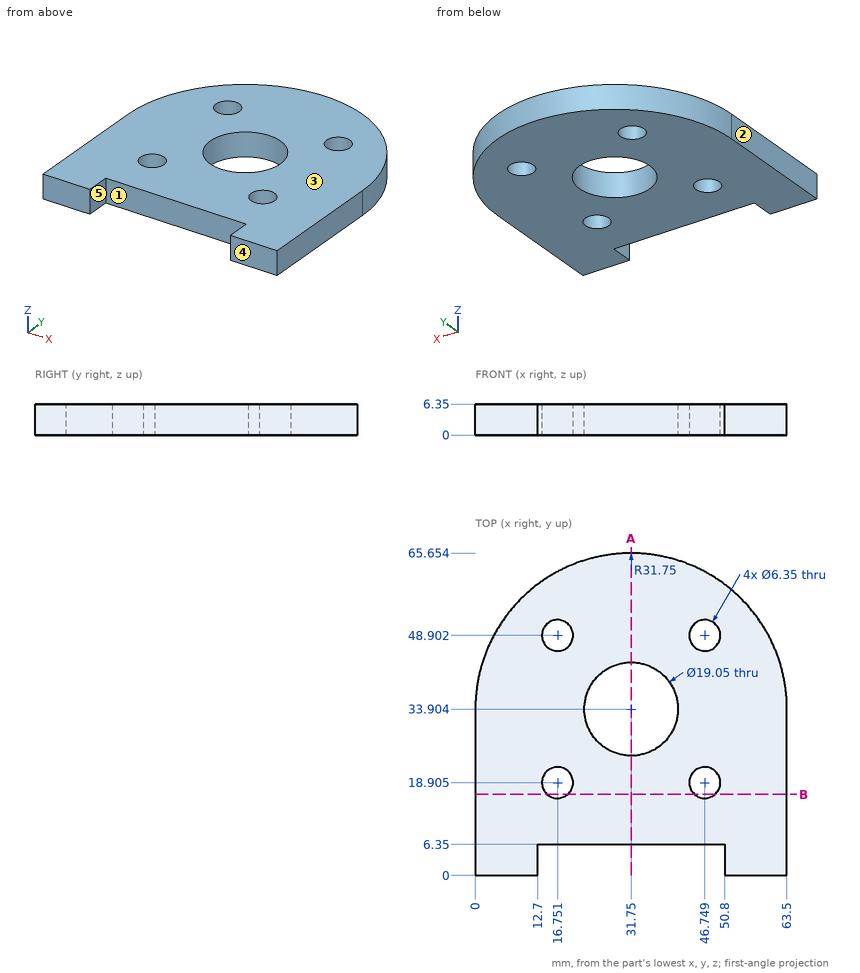
Answer from the drawing. Dimensions are ordinates in mm from the lowest x, y and z of the part. A direction names the side the tool comes from. Round coordinates to 2 decimals unless told otherwise and drop trailing zeros. Order: outer loops, then holes, each group sorted by start corner. A loop starts at its lowest first (then second) coordinate and runs counter-clockwise, first axis right, second up. Notation, with made-up numbers: (-3.5, 33) - (4.5, 33) arc R16 ccw to (4.5, 61) - close; hole circle Ø4 at (-7.75, -37.75). An arc over 180 degrees is marked (long way). Put each result on its own line as item: value. Start each with the question number.
(1) For the marked faces 4 and 5, determine the directions among +Z, -Z, +X, -X, +Y, -Y from which every point of the face is accessible in a straight line to the end or side of a thin tool.
(2) Determine the mould class of the marked faces 1, 2 and 3 for opening direction X: released by +X, released by -X, zero draft, split by the parting line, or undercut.
(3) Straight lines are drawn through the part: probe 1 along X at (y, z) = (3.5, 5.25); probe 2 along X at (y, z) = (29, 6) (1 decimal); probe 3 along Y at (x, z) = (55, 4) (1 decimal). For each, find the intervals that lie inside material, in ascending order. Write a range as from..to.
(4) Find section A-A (x = 31.75). Give the vertices of the cut face in (y, z), plus the area to 3 significant figures.
(5) Given P1, Ø17, axis at x = 31.75, y = 33.9, coming from the -Z side, flat-ended and moving along its own axis, determine where the tip first touches the part or whether it passes through.
(6) Find section B-B (y = 16.5). State how many separate pieces and enclosed holes the cut face has.
Reply:
1. face 4: +Z, -Z, +X, -X, -Y
1. face 5: +Z, -Z, -Y
2. face 1: undercut
2. face 2: released by -X
2. face 3: zero draft
3. probe 1: 0..12.7, 50.8..63.5
3. probe 2: 0..23.6, 39.9..63.5
3. probe 3: 0..55.5
4. outline: (6.35, 0) - (24.38, 0) - (24.38, 6.35) - (6.35, 6.35) - close; (43.43, 0) - (65.65, 0) - (65.65, 6.35) - (43.43, 6.35) - close
4. area: 256 mm^2
5. P1: through
6. separate pieces: 3
6. enclosed holes: 0
